Verification items for the finished model (mm, model axes). Face numbers are marked on the shaded views. A direction names the side the tool comes from. Coordinates: 2 decimals unless noted, no trailing zeros. Order: outer loops, then holes, each group sorted by start corner. A loop starts at its lowest first (then second) coordinate and runs counter-clockwise, first axis right, second up.
Q1. Cross-section at C-C, the plane z = 6.35. Record the boundary of the cut face in (x, y) (1 decimal).
Q2. Set-up check for the marked faces 4, 5 and 6: record each of +Z, -Z, +X, -X, +Y, -Y from which the full face is reachable in a straight line by a thin tool's end or side.
Q3. Cross-section at D-D, the plane y = 19. Record the boundary of the cut face in (x, z) (3 decimals).
Q4. Depth check by flat-ended pin: P1, Ø3, axis at y = 1, z = 5, coming from the +X side; P2, Ø4, axis at x = -1, y = -20.5, coming from the +Z side; P3, Ø15, axis at x = 0, y = 0, coming from the +Z side; P4, Ø4, axis at y = 6, z = 6, coming from the +X side. Enter the tip coordinate at first touch or a pass-through.
Q5. Cross-section at A-A, the plane y = 0. Record the boundary of the cut face in (x, z) (1 decimal), and give its area (3 significant figures).
Q6. Cross-section at B-B, the plane x = 0. Record the boundary of the cut face in (y, z), and give its area (3 significant figures).
Q7. Thickness scan on line 1 (X direction, y = 0, z = 3); line 2 (Y direction, x = 0, z = 3.75); line 3 (X direction, y = 0, z = 6). Record the ranges inside material, lowest first.
Q8. Draft check along X on the marked faces 1, 2 and 3. Enter one of: pulls with the +X half, pulls with the -X half, needs draft (parallel to the pull), parting line crosses it, or undercut.
from build123d import *

# Parameters (mm, degrees)
F0_W     = 76.2
F0_H     = 50.8
F0_R     = 12.7
F1_DEPTH = 12.7
F2_W     = 6.35
F2_H     = 50.8
F3_DEPTH = 2.54
F5_DEPTH = 50.8
F6_R     = 4.445
F7_DEPTH = 12.7
F8_R     = 1.5875
F9_DEPTH = 5.08


with BuildPart() as f1:
    # F0 (on Top) → F1 (new body)
    with BuildSketch(Plane.XY):
        Rectangle(F0_W, F0_H)
        Circle(F0_R, mode=Mode.SUBTRACT)
    extrude(amount=F1_DEPTH)

    # F2 (on face) → F3 (cut)
    with BuildSketch(Plane.XY.offset(12.7)):
        with Locations((-31.75, 0)):
            Rectangle(F2_W, F2_H)
        with BuildLine():
            Line((-6.35, -10.9985226281), (-6.35, -25.4))
            Line((-6.35, -25.4), (6.35, -25.4))
            Line((6.35, -25.4), (6.35, -10.9985226281))
            ThreePointArc((6.35, -10.9985226281), (0, -12.7), (-6.35, -10.9985226281))
        make_face()
        with BuildLine():
            Line((6.35, 25.4), (-6.35, 25.4))
            Line((-6.35, 25.4), (-6.35, 10.9985226281))
            ThreePointArc((-6.35, 10.9985226281), (0, 12.7), (6.35, 10.9985226281))
            Line((6.35, 10.9985226281), (6.35, 25.4))
        make_face()
    extrude(amount=-F3_DEPTH, mode=Mode.SUBTRACT)

    # F4 (on face) → F5 (cut, through all)
    with BuildSketch(Plane.XZ.offset(25.4)):
        Polygon((22.225, 12.7), (9.525, 12.7), (6.5920606325, 7.62), (25.1579393675, 7.62), align=None)
    extrude(amount=-F5_DEPTH, mode=Mode.SUBTRACT)

    # F6 (on face) → F7 (join)
    with BuildSketch(Plane.YZ.offset(38.1)):
        with Locations((0, 6.35)):
            Circle(F6_R)
    extrude(amount=F7_DEPTH)

    # F8 (on face) → F9 (join)
    with BuildSketch(Plane.YZ.offset(50.8)):
        with Locations((0, 6.35)):
            Circle(F8_R)
    extrude(amount=F9_DEPTH)


solid = f1.part
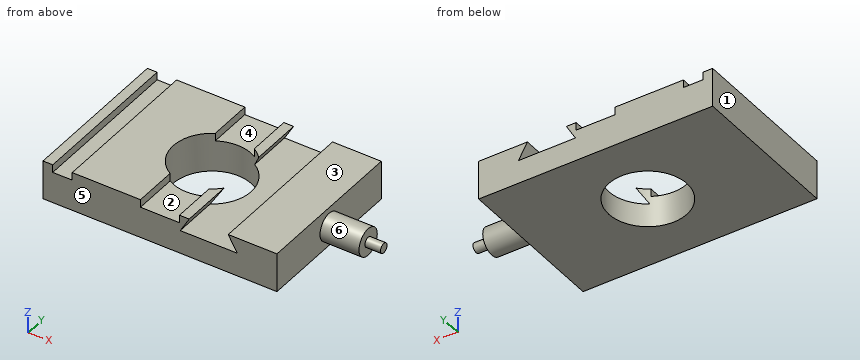
Check values:
1. outline: (-38.1, -25.4) - (38.1, -25.4) - (38.1, -4.4) - (50.8, -4.4) - (50.8, -1.6) - (55.9, -1.6) - (55.9, 1.6) - (50.8, 1.6) - (50.8, 4.4) - (38.1, 4.4) - (38.1, 25.4) - (-38.1, 25.4) - close; hole circle Ø25.4 at (0, 0)
2. face 4: +Z, +Y, -Y
2. face 5: +Z, -Z, +X, -X, -Y
2. face 6: +X
3. outline: (-38.1, 0) - (38.1, 0) - (38.1, 12.7) - (22.225, 12.7) - (25.158, 7.62) - (6.592, 7.62) - (9.525, 12.7) - (6.35, 12.7) - (6.35, 10.16) - (-6.35, 10.16) - (-6.35, 12.7) - (-28.575, 12.7) - (-28.575, 10.16) - (-34.925, 10.16) - (-34.925, 12.7) - (-38.1, 12.7) - close
4. P1: stops at x = 55.88
4. P2: stops at z = 10.16
4. P3: passes through
4. P4: stops at x = 50.8
5. outline: (-38.1, 0) - (-12.7, 0) - (-12.7, 12.7) - (-28.6, 12.7) - (-28.6, 10.2) - (-34.9, 10.2) - (-34.9, 12.7) - (-38.1, 12.7) - close; (12.7, 0) - (38.1, 0) - (38.1, 1.9) - (50.8, 1.9) - (50.8, 4.8) - (55.9, 4.8) - (55.9, 7.9) - (50.8, 7.9) - (50.8, 10.8) - (38.1, 10.8) - (38.1, 12.7) - (22.2, 12.7) - (25.2, 7.6) - (12.7, 7.6) - close
5. area: 702 mm2
6. outline: (-25.4, 0) - (-12.7, 0) - (-12.7, 10.16) - (-25.4, 10.16) - close; (12.7, 0) - (25.4, 0) - (25.4, 10.16) - (12.7, 10.16) - close
6. area: 258 mm2
7. line 1: x = -38.1 to -12.7, 12.7 to 50.8
7. line 2: y = -25.4 to -12.7, 12.7 to 25.4
7. line 3: x = -38.1 to -12.7, 12.7 to 55.88
8. face 1: pulls with the -X half
8. face 2: undercut
8. face 3: needs draft
